Here's how the part is built. I have some questions about the finished solid (model axes, mm). Face numbers are marked on the shaded views. A direction names the side the tool comes from. Round coordinates to 2 decimals unless told otherwise and drop trailing zeros. Write each loop counter-clockwise with the first axis right and the second up, starting at its lowest first coordinate (ties: lowest second). Pieces come first, ordered by that corner, then holes. Notation, with made-up numbers: (12, -22.5) -> (70, -22.5) arc R21 ccw to (70, 3.5) -> close; hole circle Ø3 at (25, 27.25). An arc over 180 degrees is marked (long way). Answer in a Markdown table with one row per item.
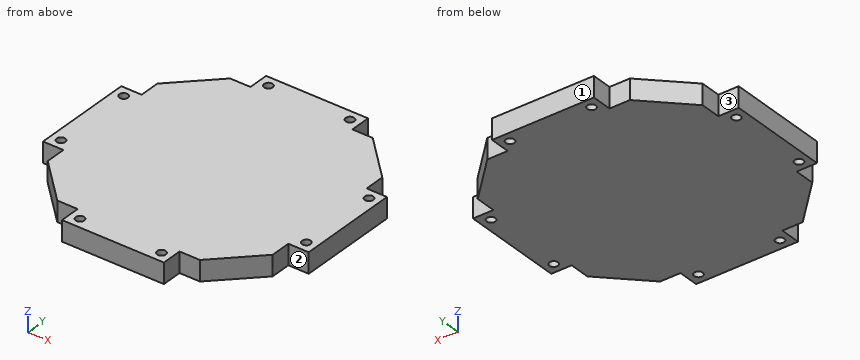
Autodesk Inventor part; units mm, degrees
ref_plane "YZ Plane" through (0, 0, 0) normal (1, 0, 0) x (0, 1, 0)
ref_plane "XZ Plane" through (0, 0, 0) normal (0, 1, 0) x (-1, 0, 0)
ref_plane "XY Plane" through (0, 0, 0) normal (0, 0, 1) x (1, 0, 0)
sketch "Sketch1" plane through (0, 0, 0) normal (0, 0, 1) x (1, 0, 0)
  line L0 (-25, 65.19) -> (25, 65.19)
  line L1 (65.19, 25) -> (65.19, -25)
  line L2 (25, -65.19) -> (-25, -65.19)
  line L3 (-65.19, -25) -> (-65.19, 25)
  line L4 (-50.6308, 50.6308) -> (50.6308, -50.6308) construction
  line L5 (50, 50) -> (-50, -50) construction
  line L6 (-40, 40) -> (-50.6308, 50.6308) construction
  line L7 (-25, 65.19) -> (-25, 55.19)
  line L8 (-25, 55.19) -> (-55.19, 55.19)
  line L9 (-55.19, 55.19) -> (-55.19, 25)
  line L10 (-55.19, 25) -> (-65.19, 25)
  line L11 (-55.19, -25) -> (-55.19, -55.19)
  line L12 (-65.19, -25) -> (-55.19, -25)
  line L13 (-55.19, -55.19) -> (-25, -55.19)
  line L14 (-25, -55.19) -> (-25, -65.19)
  line L15 (-40, -40) -> (-50.6308, -50.6308) construction
  line L16 (25, -55.19) -> (55.19, -55.19)
  line L17 (25, -65.19) -> (25, -55.19)
  line L18 (55.19, -55.19) -> (55.19, -25)
  line L19 (55.19, -25) -> (65.19, -25)
  line L20 (40, -40) -> (50.6308, -50.6308) construction
  line L21 (55.19, 25) -> (55.19, 55.19)
  line L22 (65.19, 25) -> (55.19, 25)
  line L23 (55.19, 55.19) -> (25, 55.19)
  line L24 (25, 55.19) -> (25, 65.19)
  line L25 (40, 40) -> (50.6308, 50.6308) construction
  line L26 (0, 0) -> (0, 26.4544)
  point P0 (-45.3154, 45.3154)
  point P1 (-45.3154, -45.3154)
  point P2 (45.3154, -45.3154)
  point P3 (45.3154, 45.3154)
  dimension "d9" = 130.38
  dimension "d17" = 360
  dimension "d19" = 10
  dimension "d24" = 10
  dimension "d39" = 50
extrude "Extrusion1" add sketch "Sketch1" along normal blind 10
chamfer "Chamfer1" distance 20.19 angle 45 4 edges at (-55.19, 55.19, 5) (55.19, 55.19, 5) (55.19, -55.19, 5) (-55.19, -55.19, 5)
sketch "Sketch3" plane through (0, 0, 10) normal (0, 0, 1) x (1, 0, 0)
  circle A0 centre (-20, 60.19) radius 2.1
  line L0 (25, 65.19) -> (-25, 65.19)
  line L1 (-25, 65.19) -> (-25, 55.19)
  line L2 (0, 0) -> (0, 11.031)
  line L3 (0, 0) -> (10.2151, 0)
  circle A1 centre (20, 60.19) radius 2.1
  circle A2 centre (-60.19, -20) radius 2.1
  circle A3 centre (-60.19, 20) radius 2.1
  circle A4 centre (20, -60.19) radius 2.1
  circle A5 centre (-20, -60.19) radius 2.1
  circle A6 centre (60.19, 20) radius 2.1
  circle A7 centre (60.19, -20) radius 2.1
  dimension "d30" = 4.2
  dimension "d31" = 5
  dimension "d32" = 5
  dimension "d35" = 360
extrude "Extrusion3" cut sketch "Sketch3" against normal through all
properties part number "gearbox_top" material "PMMA Plastic"
1) I want a section at A-A, the plane y = 60.19. List the corners of the cut face in (x, z) for me.
Response:
| item | result |
|---|---|
| outline | (-25, 0) -> (-22.1, 0) -> (-22.1, 10) -> (-25, 10) -> close; (-17.9, 0) -> (17.9, 0) -> (17.9, 10) -> (-17.9, 10) -> close; (22.1, 0) -> (25, 0) -> (25, 10) -> (22.1, 10) -> close |
2) I need wall thicknesses on line 1 (Y direction, x = 60.19, z = 5.5); line 2 (Y direction, x = -20, z = 3.5); line 3 (X direction, y = 59.5, z = 2.5). Which ranges of each line are inside material? Lowest first, please. Write a range as [from, to].
Response:
| item | result |
|---|---|
| line 1 | y = [-25, -22.1], [-17.9, 17.9], [22.1, 25] |
| line 2 | y = [-65.19, -62.29], [-58.09, 58.09], [62.29, 65.19] |
| line 3 | x = [-25, -21.98], [-18.02, 18.02], [21.98, 25] |
3) Which directions (+Z, -Z, +X, -X, +Y, -Y) give clear straight access to the entire face, cutting with the end or side of a thin tool? Please do the marked faces 1, 2 and 3.
Response:
| item | result |
|---|---|
| face 1 | +Z, -Z, +X, -X, +Y |
| face 2 | +Z, -Z, +X, -Y |
| face 3 | +Z, -Z, -X, +Y |
4) I want a section at C-C, the plane z = 8.25. Count the separate pieces of the cut face and the enclosed holes in it, and give its area (3 significant figures).
Response:
| item | result |
|---|---|
| separate pieces | 1 |
| enclosed holes | 8 |
| area | 13,300 mm^2 |
5) I want a section at D-D, the plane x = 49. List the corners of the cut face in (y, z) for me.
Response:
| item | result |
|---|---|
| outline | (-41.19, 0) -> (41.19, 0) -> (41.19, 10) -> (-41.19, 10) -> close |
6) For pin 1 (5.5 mm diameter, centred on x = -60.19, y = -20, fed in from +Z); pin 2 (5 mm diameter, centred on y = -60.5, z = 5, fed in from -X); pin 3 (3 mm diameter, centred on x = -30.5, z = 4.5, fed in from -Y); pin 4 (4 mm diameter, centred on x = 60.19, y = 20, fed in from +Z), each with a flat end and sliding along its axis, tell me the tip position at first contact or that it passes through.
Response:
| item | result |
|---|---|
| pin 1 | stops at z = 10 |
| pin 2 | stops at x = -25 |
| pin 3 | stops at y = -55.19 |
| pin 4 | passes through |
